Source: three-view drawing plus pictorial views. Frame: mm from the lowest corner of the part. Round coordinates to 2 decimals unless told otherwise and drop trailing zeros. Loops run counter-clockwise (first coordinate to the right, second up) from the corner with the lowest first, then second, coordinate; pieces in that order, holes last. Notation, with made-up numbers: (59, 51) -> (115, 51) arc R30 cw to (115, 85) -> close; hole circle Ø3 at (37, 3). An arc over 180 degrees is marked (long way). Answer as a JSON object with one key per item and string values. Group by question number.
Item 1: Draft query along Y for the marked faces 1, 2 and 3. Return one class per face: released by +Y, released by -Y, zero draft, split by the parting line, or undercut.
Item 2: Section query C-C on z = 26.5. Return loops of the section in (x, y).
Item 3: Pin query (flat end, axial travel): pin 1 (12 mm diameter, centred on y = 16.5, z = 12.5, fed in from -X); pin 2 (1.5 mm diameter, centred on x = 3, y = 22.5, fed in from -Z); pin 3 (3 mm diameter, centred on x = 3.5, z = 30.5, fed in from +Y). Return the tip coordinate at first contact, or that it passes through.
Item 4: Material intervals for line 1 (Y direction, x = 4.45, z = 17); line 2 (Y direction, x = 4.55, z = 17.5) (1 decimal); line 3 (Y direction, x = 4.2, z = 5.5) (1 decimal), sorted ascending. Write a range as [from, to].
Item 5: Section query D-D on x = 5.05. Count the separate pieces of the cut face and the enclosed holes in it.
Item 6: Section query A-A on y = 17. Return loops of the section in (x, z), and give its area (3 significant figures).
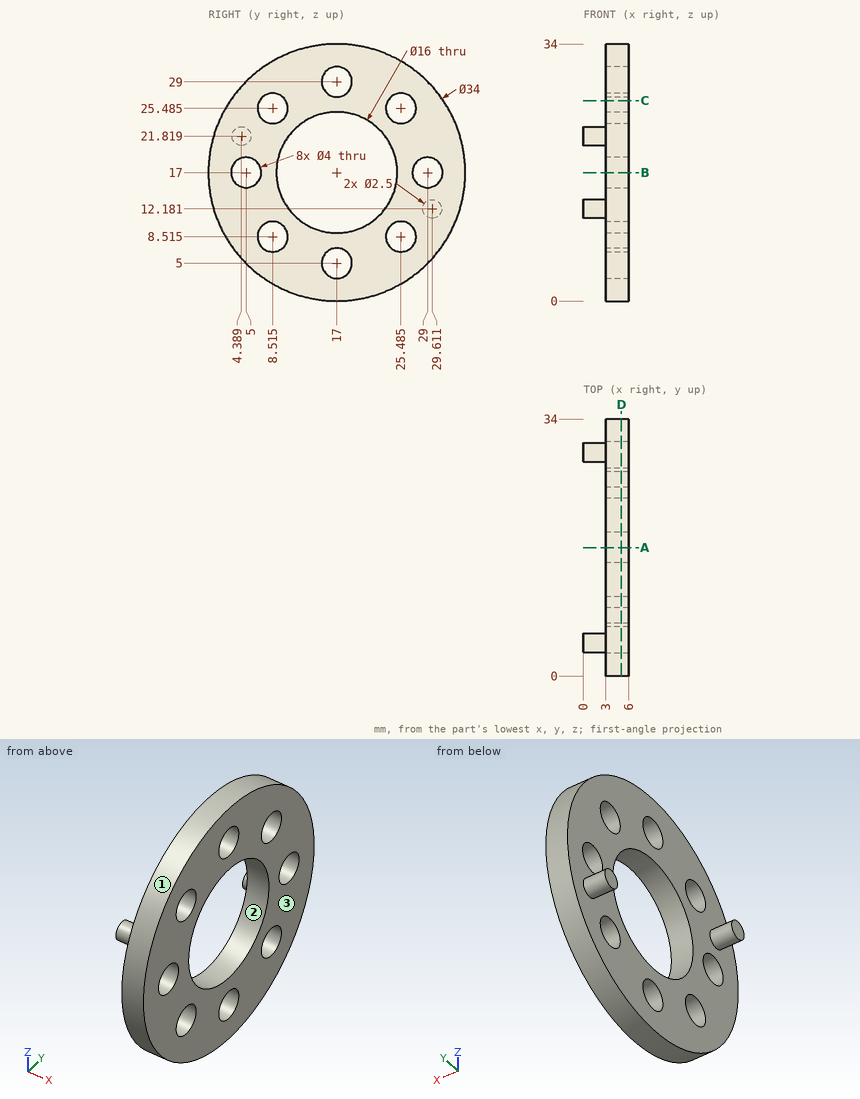
Solved:
{
 "1": {"face 1": "split by the parting line", "face 2": "undercut", "face 3": "zero draft"},
 "2": {"outline": "(3, 2.9) -> (6, 2.9) -> (6, 6.79) -> (3, 6.79) -> close; (3, 10.24) -> (6, 10.24) -> (6, 23.76) -> (3, 23.76) -> close; (3, 27.21) -> (6, 27.21) -> (6, 31.1) -> (3, 31.1) -> close"},
 "3": {"pin 1": "x = 3", "pin 2": "z = 0.68", "pin 3": "y = 29.04"},
 "4": {"line 1": "[0, 3], [7, 9], [25, 27], [31, 34]", "line 2": "[0, 3.1], [6.9, 9], [25, 27.1], [30.9, 34]", "line 3": "[4.5, 15.1], [18.9, 29.5]"},
 "5": {"separate pieces": "1", "enclosed holes": "9"},
 "6": {"outline": "(3, 0) -> (6, 0) -> (6, 3) -> (3, 3) -> close; (3, 7) -> (6, 7) -> (6, 9) -> (3, 9) -> close; (3, 25) -> (6, 25) -> (6, 27) -> (3, 27) -> close; (3, 31) -> (6, 31) -> (6, 34) -> (3, 34) -> close", "area": "30.0 mm²"}
}
